Build history of the part. All positions in model axes, mm. Face numbers are marked on the shaded views. A direction names the side the tool comes from. Round coordinates to 2 decimals unless told otherwise and drop trailing zeros. Write each loop counter-clockwise with the first axis right and the second up, starting at its lowest first coordinate (ties: lowest second). Pieces come first, ordered by that corner, then holes. Notation, with made-up numbers: M -35.5,76 L -5.5,76 A8 ccw -5.5,89 Z; hole C 54.25,33.25 d4. An arc over 180 degrees is marked long. One line per item, written item: value. Start each with the question number.
```python
from build123d import *

# Parameters (mm, degrees)
F2_DEPTH       = 10.6500000106
F4_W           = 19.24
F4_H           = 27.4
F5_DEPTH       = 2.4
F6_W           = 6
F6_H           = 0.6600641444
F7_DEPTH       = 10.6500000106
F8_W           = 19.24
F8_H           = 13.0500000106
F9_DEPTH       = 2
F10_R          = 1.95
F11_DEPTH      = 4.2
F12_W          = 6
F12_H          = 4.3
F13_DEPTH      = 3
F14_R          = 8
F15_W          = 6.6
F15_H          = 1
F16_DEPTH      = 8
F16_DEPTH_BACK = 8
F17_R          = 0.3
F18_W          = 1.5
F18_H          = 1.5
F19_DEPTH      = 5.175
F19_DEPTH_BACK = 1
F20_R          = 0.5


with BuildPart() as f2:
    # F1 (on Front) → F2 (new body)
    with BuildSketch(Plane.XZ):
        Polygon((9.62, -1), (9.62, 12.7), (7.62, 12.7), (7.62, 5.715), (7.62, 4.7), (7.62, -1), align=None)
        with BuildLine():
            Line((7.62, 5.715), (7.62, 12.7))
            Line((7.62, 12.7), (-7.62, 12.7))
            Line((-7.62, 12.7), (-7.62, 5.715))
            ThreePointArc((-7.62, 5.715), (0, 9.525), (7.62, 5.715))
        make_face()
        Polygon((-7.62, 5.715), (-7.62, 12.7), (-9.62, 12.7), (-9.62, -1), (-7.62, -1), (-7.62, 4.7), align=None)
    extrude(amount=F2_DEPTH)

    # F3: F2 across face


with BuildPart() as f2_1:
    add(f2.part)
    add(f2.part.mirror(Plane(origin=(-8.62, -5.3250000053, -1), x_dir=(1, 0, 0), z_dir=(0, 0, -1))))

    # F4 (on face) → F5 (join)
    with BuildSketch(Plane(origin=(0, 0, 0), x_dir=(-1, 0, 0), z_dir=(0, 1, 0))):
        with Locations((0, -1)):
            Rectangle(F4_W, F4_H)
    extrude(amount=F5_DEPTH)

    # F6 (on face) → F7 (cut, through all)
    with BuildSketch(Plane.XZ.offset(10.6500000106)):
        with Locations((0, -11.1949679278)):
            Rectangle(F6_W, F6_H)
    extrude(amount=-F7_DEPTH, mode=Mode.SUBTRACT)

    # F8 (on face) → F9 (join)
    with BuildSketch(Plane(origin=(0, 0, -14.7), x_dir=(1, 0, 0), z_dir=(0, 0, -1))):
        with Locations((0, 4.1250000053)):
            Rectangle(F8_W, F8_H)
    extrude(amount=F9_DEPTH)

    # F10 (on face) → F11 (cut)
    with BuildSketch(Plane.XY.offset(-11.525)):
        with Locations((0, -3)):
            Circle(F10_R)
    extrude(amount=-F11_DEPTH, mode=Mode.SUBTRACT)

    # F12 (on face) → F13 (cut)
    with BuildSketch(Plane.XY.offset(-11.525)):
        with Locations((0, -8.5000000106)):
            Rectangle(F12_W, F12_H)
    extrude(amount=-F13_DEPTH, mode=Mode.SUBTRACT)

    # F14
    f14_edges = [f2_1.edges().sort_by_distance(p)[0] for p in [
        (9.62, -4.125, 12.7),
    ]]
    fillet(f14_edges, radius=F14_R)

    # F15 (on face) → F16 (cut, two sides)
    with BuildSketch(Plane.XY.offset(-14.525)) as f16_sk:
        with Locations((0, -8.5000000106)):
            Rectangle(F15_W, F15_H)
    extrude(amount=-F16_DEPTH, mode=Mode.SUBTRACT)
    extrude(f16_sk.sketch, amount=F16_DEPTH_BACK, mode=Mode.SUBTRACT)

    # F17
    f17_edges = [f2_1.edges().sort_by_distance(p)[0] for p in [
        (3.3, -8, -13.817539),
        (-3.3, -8, -13.817539),
        (-3.3, -9, -13.817539),
        (3.3, -9, -13.817539),
    ]]
    fillet(f17_edges, radius=F17_R)

    # F18 (on face) → F19 (cut, two sides)
    with BuildSketch(Plane.XY.offset(-11.525)) as f19_sk:
        with Locations((2.55, -1)):
            Rectangle(F18_W, F18_H)
        with Locations((-2.55, -1)):
            Rectangle(F18_W, F18_H)
    extrude(amount=-F19_DEPTH, mode=Mode.SUBTRACT)
    extrude(f19_sk.sketch, amount=F19_DEPTH_BACK, mode=Mode.SUBTRACT)

    # F20
    f20_edges = [f2_1.edges().sort_by_distance(p)[0] for p in [
        (3.3, -0.25, -13.817539),
        (3.3, -1.75, -13.817539),
        (1.8, -1.75, -14.1125),
        (1.8, -0.25, -14.1125),
        (-3.3, -0.25, -13.817539),
        (-1.8, -0.25, -14.1125),
        (-1.8, -1.75, -14.1125),
        (-3.3, -1.75, -13.817539),
    ]]
    fillet(f20_edges, radius=F20_R)


solid = f2_1.part
```
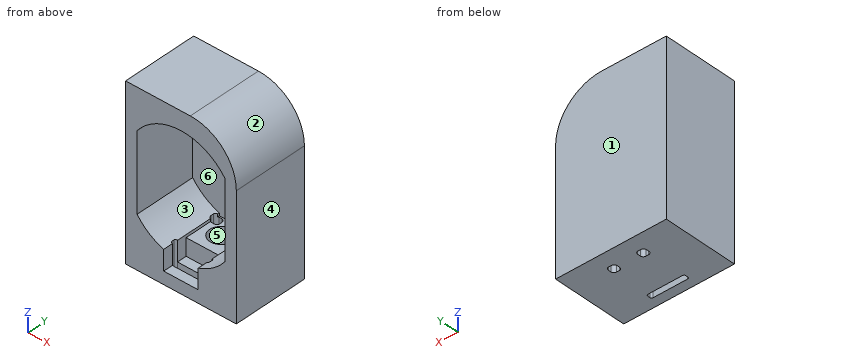
Item 1: Two-plate mould, pull along X, no slides. Class the marked faces 1, 2 and 3: pulls with the +X half, pulls with the -X half, needs draft (parallel to the pull), parting line crosses it, or undercut.
Item 2: Cut at B-B, the plane y = -7.5. Write the cut outline in (x, z) (3 decimals).
Item 3: Cut at A-A, the plane x = 0. Write the cut outline in (y, z) (3 decimals).
Item 4: Cut at D-D, the plane y = -3. Write the cut outline in (x, z) (3 decimals), plus the area to 3 significant figures.
Item 5: Drill centre lines: line 1 (Y direction, x = 0, z = -13.5); line 2 (X direction, y = -1.5, z = 2.5); line 3 (Z direction, x = 5.5, y = -1.5). Where is each one in solid material? Low to high.
Item 6: Which spindle directions (+Z, -Z, +X, -X, +Y, -Y) get a long thin tool onto all of the face, cutting with end or side? Do the marked faces 4, 5 and 6. Say none if no direction does.
Item 7: Drop a flat-ended pin along its axis: pin 1 (5 mm diameter, centred on x = 3.5, z = 4, fed in from -Y). Give the stop position or say it passes through.
Item 8: Cut at C-C, the plane z = -4. Write the cut outline in (x, y), plus the area to 3 significant figures.
Computed values:
1. face 1: needs draft
1. face 2: pulls with the +X half
1. face 3: undercut
2. outline: M -9.62,-16.7 L 9.62,-16.7 L 9.62,4.7 A8 ccw 1.62,12.7 L -9.62,12.7 Z; hole M -7.62,-7.715 A9.525 ccw -3,-11.04 L -3,-14.525 L 3,-14.525 L 3,-11.04 A9.525 ccw 7.62,-7.715 L 7.62,5.715 A9.525 ccw -7.62,5.715 Z
3. outline: M -10.65,-16.7 L -9,-16.7 L -9,-14.525 L -10.65,-14.525 Z; M -10.65,9.525 L 0,9.525 L 0,-11.525 L -1.05,-11.525 L -1.05,-15.725 L -4.95,-15.725 L -4.95,-11.525 L -6.35,-11.525 L -6.35,-14.525 L -8,-14.525 L -8,-16.7 L 2.4,-16.7 L 2.4,12.7 L -10.65,12.7 Z
4. outline: M -9.62,-16.7 L 9.62,-16.7 L 9.62,4.7 A8 ccw 1.62,12.7 L -9.62,12.7 Z; hole M -7.62,-7.715 A9.525 ccw -3,-11.04 L -3,-11.525 L -1.95,-11.525 L -1.95,-15.725 L 1.95,-15.725 L 1.95,-11.525 L 3,-11.525 L 3,-11.04 A9.525 ccw 7.62,-7.715 L 7.62,5.715 A9.525 ccw -7.62,5.715 Z
4. area: 249 mm2
5. line 1: y = -6.35 to -4.95, -1.05 to 2.4
5. line 2: x = -9.62 to -7.62, 7.62 to 9.62
5. line 3: z = -16.7 to -9.78, 7.78 to 11.7
6. face 4: +Z, -Z, +X, +Y, -Y
6. face 5: none
6. face 6: -Y
7. pin 1: stops at y = 0
8. outline: M -9.62,-10.65 L -7.62,-10.65 L -7.62,0 L 7.62,0 L 7.62,-10.65 L 9.62,-10.65 L 9.62,2.4 L -9.62,2.4 Z
8. area: 88.8 mm2
